Autodesk Inventor part; units mm, degrees
ref_plane "YZ Plane" through (0, 0, 0) normal (1, 0, 0) x (0, 1, 0)
ref_plane "XZ Plane" through (0, 0, 0) normal (0, 1, 0) x (-1, 0, 0)
ref_plane "XY Plane" through (0, 0, 0) normal (0, 0, 1) x (1, 0, 0)
sketch "Sketch1" plane through (0, 0, 0) normal (0, 0, 1) x (1, 0, 0)
  line L0 (-65, -40) -> (65, -40)
  line L1 (65, -40) -> (65, 40)
  line L2 (65, 40) -> (-65, 40)
  line L3 (-65, 40) -> (-65, -40)
  line L4 (-65, -40) -> (65, 40) construction
  line L5 (65, -40) -> (-65, 40) construction
  point P0 (0, 0)
  dimension "d0" = 80
  dimension "d1" = 130
extrude "Extrusion1" add sketch "Sketch1" along normal blind 30
sketch "Sketch2" plane through (0, 0, 30) normal (0, 0, 1) x (1, 0, 0)
  line L0 (-65, -40) -> (65, -40)
  line L1 (65, -40) -> (65, 40)
  line L2 (65, 40) -> (-65, 40)
  point P0 (0, 0)
  point P1 (0, 40)
hole "Hole1" at (0, 40, 30) direction (0, 0, -1) diameter 9 depth 30
chamfer "Chamfer1" distance 5 angle 45 5 edges at (34.75, 40, 30) (-34.75, 40, 30) (65, 0, 30) (0, -40, 30) (-65, 0, 30)
properties part number "block"
Could you check a few things on this model? Use its own coordinates, in mm. Coordinates: 2 decimals unless noted, no trailing zeros. Write each loop counter-clockwise with the first axis right and the second up, starting at its lowest first coordinate (ties: lowest second). Pieces come first, ordered by that corner, then holes. Notation, with made-up numbers: (64.25, 35) -> (92.25, 35) arc R32 cw to (92.25, 68) -> close; hole circle Ø7 at (50, 69.25). An arc over 180 degrees is marked (long way). One line per question, with ' | ' between items. Start each with the question number.
1. If we section it at A-A (x = 0): Please give me the cut outline in (y, z), and give its area (3 significant figures).
2. Will this pin go through, and if not, where does the flat tip stop? P1, Ø8, axis at x = -38.5, y = 30, coming from the -Z side.
3. Thinking about a two-plate mould opening in X: for faces 1 (the face through (0.1, 35.5, 14.6)), 2 (the face through (-1, 1, 0)), 3 (the face through (65, -1, 12)), which applies, pulls with the +X half, pulls with the -X half, needs draft (parallel to the pull), parting line crosses it, or undercut?
4. Please list where these lines run through material, in increasing order: line 1 along X through (y, z) = (37, 12); line 2 along X through (y, z) = (-12.5, 28).
Return value:
1) outline: (-40, 0) -> (35.5, 0) -> (35.5, 29.5) -> (35, 30) -> (-35, 30) -> (-40, 25) -> close | area: 2,250 mm²
2) P1: stops at z = 0
3) face 1: undercut | face 2: needs draft | face 3: pulls with the +X half
4) line 1: x = -65 to -3.35, 3.35 to 65 | line 2: x = -62 to 62
